Geometry: final body of the model. Coordinates: model frame, mm. Coordinates: 2 decimals unless noted, no trailing zeros. Loops run counter-clockwise (first coordinate to the right, second up) from the corner with the lowest first, then second, coordinate; pieces in that order, holes last. Notation, with made-up numbers: (60, -24) - (64, -24) arc R24 cw to (64, 2) - close; hole circle Ø1 at (52.25, -13.75). An arc over 180 degrees is marked (long way). Put each result on its own line as item: value. Start each with the question number.
1) Section A-A on x = 0. Output: boundary loops of the cut face in (y, z), and give its area (3 significant figures).
2) Section B-B on z = 0. Output: boundary loops of the cut face in (x, y) (3 decimals).
3) Contact query for flat-ended pins moving along their axis: pin 1 Ø5.5 at (y, z) = (10.5, 3) entering from -X; pin 2 Ø2.5 at (y, z) = (1, -65.5) entering from -X; pin 3 Ø4 at (x, z) = (-95, 93.5) entering from +Y. Output: stop coordinate, or through.
4) Material intervals for line 1 along X through (y, z) = (10.5, -9.5); line 2 along Z through (x, y) = (94, 0.6); line 3 along Y through (x, z) = (24, -85), sorted ascending. Write a range as from..to.
5) Section C-C on y = 10.5. Output: boundary loops of the cut face in (x, z).
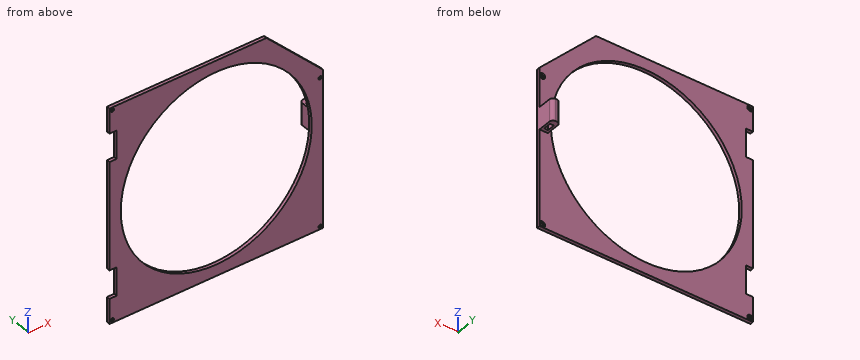
Autodesk Inventor part; units mm, degrees
ref_plane "YZ Plane" through (0, 0, 0) normal (1, 0, 0) x (0, 1, 0)
ref_plane "XZ Plane" through (0, 0, 0) normal (0, 1, 0) x (-1, 0, 0)
ref_plane "XY Plane" through (0, 0, 0) normal (0, 0, 1) x (1, 0, 0)
sketch "Sketch1" plane through (0, 0, 0) normal (0, 1, 0) x (-1, 0, 0)
  line L0 (101.6, -101.6) -> (-101.6, -101.6)
  line L1 (-101.6, -101.6) -> (-101.6, 101.6)
  line L2 (-101.6, 101.6) -> (101.6, 101.6)
  line L3 (101.6, 101.6) -> (101.6, -101.6)
  line L4 (96.6, -96.6) -> (-96.6, -96.6)
  line L5 (-96.6, -96.6) -> (-96.6, 96.6)
  line L6 (-96.6, 96.6) -> (96.6, 96.6)
  line L7 (96.6, 96.6) -> (96.6, -96.6)
  line L8 (101.6, 101.6) -> (-40.4, 101.6)
  circle A0 centre (0, 0) radius 86.4
  circle A1 centre (0, 0) radius 109.3376
  line L9 (-40.4, 101.6) -> (-101.6, 40.4)
  line L10 (-45.4, 101.6) -> (-101.6, 45.4)
  line L11 (96.6, 96.6) -> (96.6, 101.6)
  line L12 (-45.4, 101.6) -> (-35.4, 101.6)
  line L13 (-35.4, 101.6) -> (-35.4, 96.6)
  line L14 (-35.4, 96.6) -> (-45.4, 96.6)
  line L15 (-45.4, 96.6) -> (-45.4, 101.6)
  circle A2 centre (0, 0) radius 111.3376
  point P0 (96.6, 51.2168)
  point P1 (101.6, 40.4)
  point P2 (101.6, -40.4)
  point P3 (96.6, -51.2168)
  point P4 (-96.6, 45.4)
  point P5 (-45.4, 96.6)
  dimension "d0" = 203.2
  dimension "d1" = 203.2
  dimension "d2" = 101.6
  dimension "d3" = 101.6
  dimension "d4" = 5
  dimension "d5" = 5
  dimension "d6" = 5
  dimension "d7" = 5
  dimension "d10" = 142
  dimension "d12" = 61.2
  dimension "d14" = 172.8
  dimension "d15" = 5
  dimension "d16" = 5
  dimension "d17" = 10
  dimension "d34" = 2
extrude "Extrusion1" add sketch "Sketch1" along normal blind 3 contours A2 L7 L4 | L4 A1 L7 A2 | L4 A1 L5 L9 L6 L7 | A2 L5 A1 L4 | L4 L5 A2 | A1 L6 A2 L7 | A2 L6 L7
sketch "Sketch5" plane through (0, 3, 0) normal (0, 1, 0) x (1, 0, 0)
  line L0 (-96.6, -96.6) -> (45.4, -96.6)
  circle A0 centre (0, 0) radius 86.4
  line L1 (96.6, -45.4) -> (96.6, 96.6)
  line L2 (96.6, 0) -> (89.1, 0)
  line L3 (89.1, 0) -> (89.1, 10)
  line L4 (89.1, 10) -> (96.6, 10)
  line L5 (96.6, 10) -> (96.6, 0)
  line L6 (89.1, 0) -> (96.6, 0)
  line L7 (96.6, 0) -> (96.6, -10)
  line L8 (96.6, -10) -> (89.1, -10)
  line L9 (89.1, -10) -> (89.1, 0)
  line L10 (0, 0) -> (96.6, 0)
  point P0 (10, -96.6)
  dimension "d52" = 7.5
  dimension "d53" = 7.5
  dimension "d54" = 10
  dimension "d55" = 10
extrude "Extrusion4" add sketch "Sketch5" along normal blind 15 contours L3 L4 L1 L2 | L2 L1 L8 L9
sketch "Sketch7" plane through (89.1, 3, 10) normal (0, 0, 1) x (1, 0, 0)
  line L0 (2, 10) -> (5.5, 10)
  line L1 (5.5, 10) -> (5.5, 3)
  line L2 (5.5, 3) -> (2, 3)
  line L3 (2, 3) -> (2, 10)
  line L4 (7.5, 0) -> (7.5, 15)
  line L5 (0, 0) -> (0, 15)
  line L6 (0, 15) -> (7.5, 15)
  point P0 (-89.1, -3)
  dimension "d56" = 3.5
  dimension "d57" = 2
  dimension "d58" = 2
  dimension "d59" = 5
  dimension "d60" = 7
extrude "Extrusion6" cut sketch "Sketch7" against normal through all
fillet "Fillet7" radius 3.175 2 edges at (96.6, 18, 0) (89.1, 18, 0)
sketch "Sketch8" plane through (0, 3, 0) normal (0, 1, 0) x (1, 0, 0)
  arc A0 (-101.6, -98.425) -> (-98.425, -101.6) centre (-98.425, -98.425) ccw
  line L0 (44.0849, 101.6) -> (-98.425, 101.6)
  line L1 (-101.6, 98.425) -> (-101.6, -98.425)
  line L2 (-101.6, -46.1) -> (-101.6, -76.6)
  line L3 (-96.6, -96.6) -> (-96.6, 96.6)
  line L4 (-96.6, -46.1) -> (-96.6, -76.6)
  line L5 (-101.6, -76.6) -> (-96.6, -76.6)
  line L6 (-101.6, -46.1) -> (-96.6, -46.1)
  line L7 (-98.425, -101.6) -> (101.6, -101.6)
  line L8 (0, 0) -> (-101.6, 0)
  line L9 (-101.6, 46.1) -> (-101.6, 76.6)
  line L10 (-96.6, 46.1) -> (-96.6, 76.6)
  line L11 (-101.6, 76.6) -> (-96.6, 76.6)
  line L12 (-101.6, 46.1) -> (-96.6, 46.1)
  line L13 (-96.6, -76.6) -> (-90.1, -76.6)
  line L14 (-90.1, -76.6) -> (-90.1, -46.1)
  line L15 (-90.1, -46.1) -> (-96.6, -46.1)
  line L16 (-96.6, -46.1) -> (-96.6, -76.6)
  arc A1 (-98.425, 101.6) -> (-101.6, 98.425) centre (-98.425, 98.425) ccw
  line L17 (-101.6, 46.1) -> (-101.6, 76.6)
  line L18 (-96.6, 46.1) -> (-96.6, 76.6)
  line L19 (-101.6, 76.6) -> (-96.6, 76.6)
  line L20 (-101.6, 46.1) -> (-96.6, 46.1)
  line L21 (-96.6, 76.6) -> (-90.1, 76.6)
  line L22 (-90.1, 76.6) -> (-90.1, 46.1)
  line L23 (-90.1, 46.1) -> (-96.6, 46.1)
  line L24 (-96.6, 46.1) -> (-96.6, 76.6)
  line L25 (-96.6, -76.6) -> (-101.6, -76.6)
  line L26 (-101.6, -76.6) -> (-101.6, -74.1)
  line L27 (-101.6, -74.1) -> (-96.6, -74.1)
  line L28 (-96.6, -74.1) -> (-96.6, -76.6)
  line L29 (-96.6, -46.1) -> (-101.6, -46.1)
  line L30 (-101.6, -46.1) -> (-101.6, -48.6)
  line L31 (-101.6, -48.6) -> (-96.6, -48.6)
  line L32 (-96.6, -48.6) -> (-96.6, -46.1)
  line L33 (-96.6, -76.6) -> (-90.1, -76.6)
  line L34 (-90.1, -76.6) -> (-90.1, -74.1)
  line L35 (-90.1, -74.1) -> (-96.6, -74.1)
  line L36 (-96.6, -74.1) -> (-96.6, -76.6)
  line L37 (-96.6, -48.6) -> (-90.1, -48.6)
  line L38 (-90.1, -48.6) -> (-90.1, -46.1)
  line L39 (-90.1, -46.1) -> (-96.6, -46.1)
  line L40 (-96.6, -46.1) -> (-96.6, -48.6)
  line L41 (-96.6, 96.6) -> (-96.6, -96.6)
  line L42 (-90.1, 46.1) -> (-96.6, 46.1)
  line L43 (-96.6, 46.1) -> (-96.6, 48.6)
  line L44 (-96.6, 48.6) -> (-90.1, 48.6)
  line L45 (-90.1, 48.6) -> (-90.1, 46.1)
  line L46 (-90.1, 76.6) -> (-96.6, 76.6)
  line L47 (-96.6, 76.6) -> (-96.6, 74.1)
  line L48 (-96.6, 74.1) -> (-90.1, 74.1)
  line L49 (-90.1, 74.1) -> (-90.1, 76.6)
  point P0 (-98.425, 98.425)
  point P1 (46.1, 101.6)
  point P2 (46.1, 96.6)
  point P3 (76.6, 96.6)
  point P4 (76.6, 101.6)
  point P5 (-46.1, 96.6)
  dimension "d64" = 30.5
  dimension "d65" = 25
  dimension "d66" = 6.5
  dimension "d118" = 2.5
  dimension "d119" = 2.5
  dimension "d120" = 2.5
  dimension "d121" = 2.5
extrude "Extrusion7" cut sketch "Sketch8" against normal through all contours L48 L22 L44 L3 | L37 L14 L35 L3
sketch "Sketch11" plane through (0, 3, 0) normal (0, 1, 0) x (1, 0, 0)
  line L0 (-94, 94) -> (94, 94)
  line L1 (94, 94) -> (94, -94)
  line L2 (94, -94) -> (-94, -94)
  line L3 (-94, -94) -> (-94, 94)
  circle A0 centre (-94, 94) radius 1.5
  circle A1 centre (94, 94) radius 1.5
  circle A2 centre (-94, -94) radius 1.5
  circle A3 centre (94, -39.0849) radius 1.5
  point P0 (0, 0)
  point P1 (0, 0)
  dimension "d98" = 94
  dimension "d99" = 94
  dimension "d100" = 94
  dimension "d101" = 94
  dimension "d102" = 3
  dimension "d103" = 3
  dimension "d104" = 3
  dimension "d105" = 3
extrude "Extrusion8" cut sketch "Sketch11" against normal blind 10 contours L3 A0 L0 | L0 A0 L3 | A1 L1 L0 | L0 L1 A1 | A2 L2 L3 | L3 L2 A2 | A3 L1 | L1 A3
sketch "Sketch12" plane through (0, 3, 0) normal (0, 1, 0) x (1, 0, 0)
  line L0 (-94, 94) -> (94, 94)
  line L1 (94, 94) -> (94, -94)
  line L2 (94, -94) -> (-94, -94)
  line L3 (-94, -94) -> (-94, 94)
  circle A0 centre (-94, 94) radius 2.6
  circle A1 centre (94, 94) radius 2.6
  circle A2 centre (-94, -94) radius 2.6
  circle A3 centre (94, -39.0849) radius 2.6
  point P0 (0, 0)
  point P1 (0, 0)
  point P2 (0, 0)
  dimension "d108" = 94
  dimension "d109" = 94
  dimension "d110" = 94
  dimension "d111" = 94
  dimension "d112" = 5.2
  dimension "d113" = 5.2
  dimension "d114" = 5.2
  dimension "d115" = 5.2
extrude "Extrusion9" cut sketch "Sketch12" against normal blind 1.5 contours L3 A0 L0 | L0 A0 L3 | A1 L1 L0 | L0 L1 A1 | A2 L2 L3 | L3 L2 A2 | A3 L1 | L1 A3
equation "\"d1\" = d0"
properties part number "Box_Walls_2"
Answer block:
1. outline: (0, -96.6) - (3, -96.6) - (3, -86.4) - (0, -86.4) - close; (0, 86.4) - (3, 86.4) - (3, 96.6) - (0, 96.6) - close
1. area: 61.2 mm²
2. outline: (-96.6, 0) - (-86.4, 0) - (-86.4, 3) - (-96.6, 3) - close; (86.4, 0) - (96.6, 0) - (96.6, 14.825) arc R3.175 ccw to (93.425, 18) - (92.275, 18) arc R3.175 ccw to (89.1, 14.825) - (89.1, 3) - (86.4, 3) - close; hole (91.1, 6) - (94.6, 6) - (94.6, 13) - (91.1, 13) - close
3. pin 1: stops at x = 89.1
3. pin 2: stops at x = -90.1
3. pin 3: stops at y = 3
4. line 1: x = 89.1..91.1, 94.6..96.6
4. line 2: z = -96.6..-95.5, -92.5..37.58, 40.58..48
4. line 3: y = 0..3
5. outline: (89.1, -10) - (91.1, -10) - (91.1, 10) - (89.1, 10) - close; (94.6, -10) - (96.6, -10) - (96.6, 10) - (94.6, 10) - close
